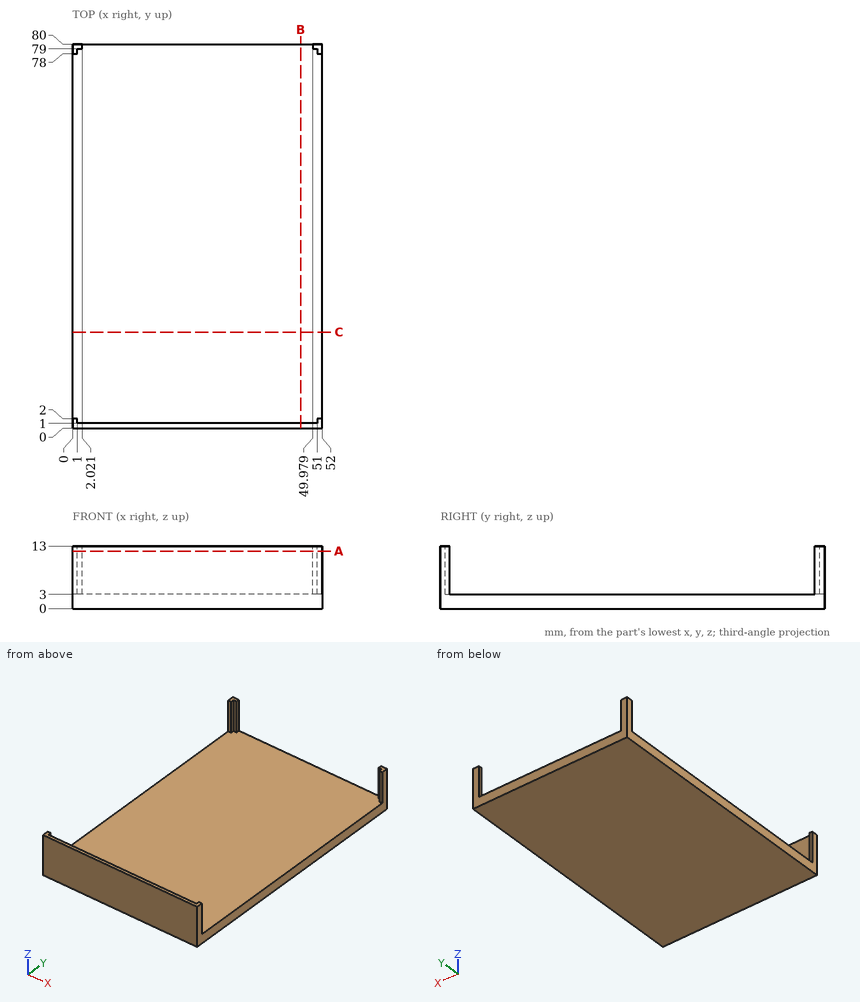
Can you work these out from the drawing? Everything is in mm from the part's minimum corner. Round coordinates to 2 decimals unless told otherwise and drop trailing zeros. Loops run counter-clockwise (first coordinate to the right, second up) from the corner with the lowest first, then second, coordinate; pieces in that order, holes last. Notation, with made-up numbers: M -23,-9.5 L 9,-9.5 A23 cw 9,18.5 Z; hole C 0,8 d11. An arc over 180 degrees is marked long. Answer in a Markdown table with one row per item.
1. If we section it at C-C, the plane y = 20: Please give me the cut outline in (x, z), plus the area to 3 significant figures.
Established:
| item | result |
|---|---|
| outline | M 0,0 L 52,0 L 52,3 L 0,3 Z |
| area | 156 mm² |
2. Please list where these lines run through material, in increasing order: line 1 (Y direction, x = 36.5, z = 5.25); line 2 (Z direction, x = 7.5, y = 29). Write a range as from..to.
Established:
| item | result |
|---|---|
| line 1 | 0..1 |
| line 2 | 0..3 |
3. If we section it at A-A, the plane z = 12: Please give me the cut outline in (x, y).
Established:
| item | result |
|---|---|
| outline | M 0,0 L 52,0 L 52,2 L 51,2 L 51,1 L 1,1 L 1,2 L 0,2 Z; M 0,78 L 1,78 L 1,79 L 2.02,79 L 2.02,80 L 0,80 Z; M 49.98,79 L 51,79 L 51,78 L 52,78 L 52,80 L 49.98,80 Z |
4. If we section it at B-B, the plane x = 47.5: Please give me the cut outline in (y, z).
Established:
| item | result |
|---|---|
| outline | M 0,0 L 80,0 L 80,3 L 1,3 L 1,13 L 0,13 Z |
5. I'm going to push flat-ended pins straight in: pin 1 Ø1.5 at (y, z) = (15, 5) entering from +X; pin 2 Ø15.5 at (x, y) = (20, 21.5) entering from +Z; pin 3 Ø3 at (x, z) = (15, 6.5) entering from +Y. Where does each tip first touch, or does it pass through?
Established:
| item | result |
|---|---|
| pin 1 | through |
| pin 2 | z = 3 |
| pin 3 | y = 1 |
